Could you check a few things on this model? Use its own coordinates, in mm. Face numbers are marked on the shaded views. A direction names the side the tool comes from. Coordinates: 2 decimals unless noted, no trailing zeros. Loops run counter-clockwise (first coordinate to the right, second up) from the corner with the lowest first, then second, coordinate; pieces in that order, holes last. Notation, with made-up numbers: (74.5, 38.5) - (86.5, 38.5) arc R17 cw to (86.5, 62.5) - close; hole circle Ø5 at (30.5, 35.5). An arc over 180 degrees is marked (long way). Use CSV: the item, a comma, the result in double quotes.
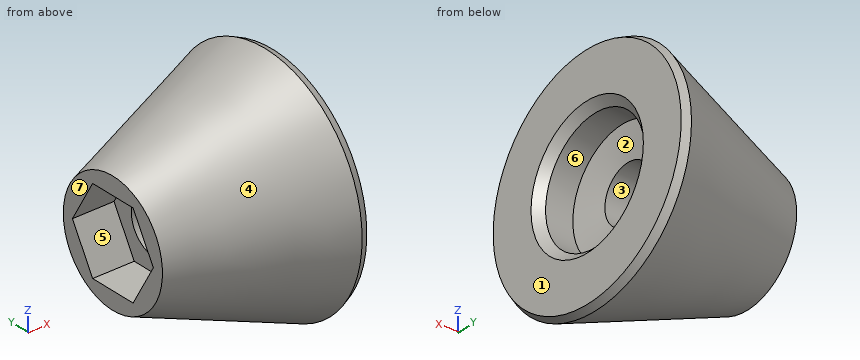
from build123d import *
from OCP.BRepFilletAPI import BRepFilletAPI_MakeChamfer

# Parameters (mm, degrees)
CORTAR_EXTRUIR1_DEPTH = 5.2
CHAFL_N1_SIZE         = 1
CHAFL_N1_SIZE2        = 0.776727613


with BuildPart() as part:
    # Croquis1 → Revolución1 (revolve)
    with BuildSketch(Plane(origin=(0, 0, 0), x_dir=(0, 1, 0), z_dir=(0, 0, 1))):
        Polygon((7.5, -10), (15, -10), (7.5, 10), (3.5, 10), (3.5, -4.894692077), (7.5, -5.6), align=None)
    revolve(axis=Axis((0, 0, 0), (-1, 0, 0)))

    # Croquis2 → Cortar-Extruir1 (cut)
    with BuildSketch(Plane(origin=(-10, 0, 0), x_dir=(0, -1, 0), z_dir=(-1, 0, 0))):
        Polygon((3.059956427, -5.3), (6.119912853, 0), (3.059956427, 5.3), (-3.059956427, 5.3), (-6.119912853, 0), (-3.059956427, -5.3), align=None)
    extrude(amount=-CORTAR_EXTRUIR1_DEPTH, mode=Mode.SUBTRACT)

    # Chaflán1: one chamfer whose edges measure the first distance from different faces: ONE call of the kernel's chamfer builder (chamfer() names one face for all edges)
    chafl_n1_edges_1 = [part.edges().sort_by_distance(p)[0] for p in [
        (10, -7.5, 0),
    ]]
    chafl_n1_edges_2 = [part.edges().sort_by_distance(p)[0] for p in [
        (10, -15, 0),
    ]]
    chafl_n1_side_2 = [part.faces().sort_by_distance(p)[0] for p in [
        (0, -11.25, 0),
    ]]
    chafl_n1 = BRepFilletAPI_MakeChamfer(part.part.solid().wrapped)
    for e in chafl_n1_edges_1:
        chafl_n1.Add(CHAFL_N1_SIZE, e.wrapped)
    for e in chafl_n1_edges_2:
        chafl_n1.Add(CHAFL_N1_SIZE, CHAFL_N1_SIZE2, e.wrapped, chafl_n1_side_2[0].wrapped)  # the first distance lies on this face
    add(Compound.cast(chafl_n1.Shape()), mode=Mode.REPLACE)


solid = part.part
(1) Will these pins go through, and if not, where does the flat tip stop? pin 1 (4 mm diameter, centred on y = 3, z = 2.5, fed in from +X); pin 2 (5.5 mm diameter, centred on x = -7.5, y = -1, fed in from +Z); pin 3 (13.5 mm diameter, centred on y = 0, z = 0, fed in from +X); pin 4 (1 mm diameter, centred on y = 0, z = -2.5, fed in from +X).
Computed:
pin 1,"stops at x = 5.32"
pin 2,"stops at z = 9.44"
pin 3,"stops at x = 5.47"
pin 4,"passes through"
(2) Thinking about a two-plate mould opening in Y: for the marked faces 1, 2, 3 and 4, which applies, +Y half, -Y half, draft (parallel to the pull), parting line (faces both ways), or undercut?
Computed:
face 1,"draft"
face 2,"undercut"
face 3,"undercut"
face 4,"parting line"
(3) Suppose I cut it at D-D (x = -4). Write out the boundary of the cut face in (y, z), plus the area to 3 significant figures.
Computed:
outline,"circle Ø19.5 at (0, 0); hole circle Ø7 at (0, 0)"
area,"260 mm²"
(4) Suppose I cut it at B-B (x = -2). Write out the boundary of the cut face in (y, z), plus the area to 3 significant figures.
Computed:
outline,"circle Ø21 at (0, 0); hole circle Ø7 at (0, 0)"
area,"308 mm²"
(5) Which directions (+Z, -Z, +X, -X, +Y, -Y) give clear straight access to the entire face, cutting with the end or side of a thin tool? Please do the marked faces 5, 6 and 7.
Computed:
face 5,"-X"
face 6,"+X"
face 7,"+Z, -Z, -X, +Y, -Y"
(6) Suppose I cut it at C-C (x = -8.5). Write out the boundary of the cut face in (y, z) (1 decimal).
Computed:
outline,"circle Ø16.1 at (0, 0); hole (-6.1, 0) - (-3.1, -5.3) - (3.1, -5.3) - (6.1, 0) - (3.1, 5.3) - (-3.1, 5.3) - close"
(7) Suppose I cut it at A-A (y = 0). Write out the boundary of the cut face in (x, z).
Computed:
outline,"(-10, -7.5) - (9.06, -14.65) - (10, -14.22) - (10, -8.5) - (9, -7.5) - (5.6, -7.5) - (4.89, -3.5) - (-4.8, -3.5) - (-4.8, -5.3) - (-10, -5.3) - close; (-10, 5.3) - (-4.8, 5.3) - (-4.8, 3.5) - (4.89, 3.5) - (5.6, 7.5) - (9, 7.5) - (10, 8.5) - (10, 14.22) - (9.06, 14.65) - (-10, 7.5) - close"
(8) Please list where these lines run through material, in increasing order: line 1 (Y direction, x = -5, z = 0.75); line 2 (Z direction, x = 6.85, y = 0); line 3 (Z direction, x = -6.75, y = 3.25).
Computed:
line 1,"y = -9.34 to -5.69, 5.69 to 9.34"
line 2,"z = -13.82 to -7.5, 7.5 to 13.82"
line 3,"z = -8.09 to -4.97, 4.97 to 8.09"
